from build123d import *

# Parameters (mm, degrees)
ESQUISSE1_R             = 52.5
BOSS_EXTRU_1_DEPTH      = 25
ESQUISSE2_R             = 40
ENL_V_MAT_EXTRU_1_DEPTH = 20
ESQUISSE3_R             = 22.3
BOSS_EXTRU_2_DEPTH      = 10
CHANFREIN1_SIZE         = 2
ENL_V_MAT_EXTRU_2_REACH = 77.746
ESQUISSE4_R             = 2
ESQUISSE4_R_2           = 6
ESQUISSE5_R             = 47.5
ESQUISSE5_R_2           = 42
ENL_V_MAT_EXTRU_3_DEPTH = 5
CONG_2_R                = 2.75
CHANFREIN2_SIZE         = 1
ESQUISSE6_R             = 5
ENL_V_MAT_EXTRU_4_DEPTH = 5


with BuildPart() as part:
    # Esquisse1 → Boss.-Extru.1 (new body)
    with BuildSketch(Plane(origin=(0, 0, 0), x_dir=(1, 0, 0), z_dir=(0, 1, 0))):
        with Locations(Location((0, 0, 0), (0, 0, 270))):
            Circle(ESQUISSE1_R)
    extrude(amount=BOSS_EXTRU_1_DEPTH)

    # Esquisse2 → Enlèv. mat.-Extru.1 (cut)
    with BuildSketch(Plane(origin=(0, 25, 0), x_dir=(1, 0, 0), z_dir=(0, 1, 0))):
        with Locations(Location((0, 0, 0), (0, 0, 270))):
            Circle(ESQUISSE2_R)
    extrude(amount=-ENL_V_MAT_EXTRU_1_DEPTH, mode=Mode.SUBTRACT)

    # Esquisse3 → Boss.-Extru.2 (add)
    with BuildSketch(Plane(origin=(0, 5, 0), x_dir=(1, 0, 0), z_dir=(0, 1, 0))):
        with Locations(Location((0, 0, 0), (0, 0, 270))):
            Circle(ESQUISSE3_R)
    extrude(amount=BOSS_EXTRU_2_DEPTH)

    # Chanfrein1
    chanfrein1_edges = [part.edges().sort_by_distance(p)[0] for p in [
        (0, 15, -22.3),
    ]]
    chamfer(chanfrein1_edges, length=CHANFREIN1_SIZE)

    # Esquisse4 → Enlèv. mat.-Extru.2 (cut, up to next)
    with BuildSketch(Plane(origin=(0, 15, 0), x_dir=(1, 0, 0), z_dir=(0, 1, 0)), mode=Mode.PRIVATE) as enl_v_mat_extru_2_sk1:
        with Locations(Location((0, 16, 0), (0, 0, 270))):
            Circle(ESQUISSE4_R)
    enl_v_mat_extru_2_tool1 = extrude(enl_v_mat_extru_2_sk1.sketch, amount=-ENL_V_MAT_EXTRU_2_REACH, mode=Mode.PRIVATE) & part.part
    # Esquisse4 → Enlèv. mat.-Extru.2 (cut, up to next)
    with BuildSketch(Plane(origin=(0, 15, 0), x_dir=(1, 0, 0), z_dir=(0, 1, 0)), mode=Mode.PRIVATE) as enl_v_mat_extru_2_sk2:
        with Locations(Location((13.856406461, 8, 0), (0, 0, 270))):
            Circle(ESQUISSE4_R)
    enl_v_mat_extru_2_tool2 = extrude(enl_v_mat_extru_2_sk2.sketch, amount=-ENL_V_MAT_EXTRU_2_REACH, mode=Mode.PRIVATE) & part.part
    # Esquisse4 → Enlèv. mat.-Extru.2 (cut, up to next)
    with BuildSketch(Plane(origin=(0, 15, 0), x_dir=(1, 0, 0), z_dir=(0, 1, 0)), mode=Mode.PRIVATE) as enl_v_mat_extru_2_sk3:
        with Locations(Location((13.856406461, -8, 0), (0, 0, 270))):
            Circle(ESQUISSE4_R)
    enl_v_mat_extru_2_tool3 = extrude(enl_v_mat_extru_2_sk3.sketch, amount=-ENL_V_MAT_EXTRU_2_REACH, mode=Mode.PRIVATE) & part.part
    # Esquisse4 → Enlèv. mat.-Extru.2 (cut, up to next)
    with BuildSketch(Plane(origin=(0, 15, 0), x_dir=(1, 0, 0), z_dir=(0, 1, 0)), mode=Mode.PRIVATE) as enl_v_mat_extru_2_sk4:
        with Locations(Location((0, -16, 0), (0, 0, 270))):
            Circle(ESQUISSE4_R)
    enl_v_mat_extru_2_tool4 = extrude(enl_v_mat_extru_2_sk4.sketch, amount=-ENL_V_MAT_EXTRU_2_REACH, mode=Mode.PRIVATE) & part.part
    # Esquisse4 → Enlèv. mat.-Extru.2 (cut, up to next)
    with BuildSketch(Plane(origin=(0, 15, 0), x_dir=(1, 0, 0), z_dir=(0, 1, 0)), mode=Mode.PRIVATE) as enl_v_mat_extru_2_sk5:
        with Locations(Location((-13.856406461, -8, 0), (0, 0, 270))):
            Circle(ESQUISSE4_R)
    enl_v_mat_extru_2_tool5 = extrude(enl_v_mat_extru_2_sk5.sketch, amount=-ENL_V_MAT_EXTRU_2_REACH, mode=Mode.PRIVATE) & part.part
    # Esquisse4 → Enlèv. mat.-Extru.2 (cut, up to next)
    with BuildSketch(Plane(origin=(0, 15, 0), x_dir=(1, 0, 0), z_dir=(0, 1, 0)), mode=Mode.PRIVATE) as enl_v_mat_extru_2_sk6:
        with Locations(Location((-13.856406461, 8, 0), (0, 0, 270))):
            Circle(ESQUISSE4_R)
    enl_v_mat_extru_2_tool6 = extrude(enl_v_mat_extru_2_sk6.sketch, amount=-ENL_V_MAT_EXTRU_2_REACH, mode=Mode.PRIVATE) & part.part
    # Esquisse4 → Enlèv. mat.-Extru.2 (cut, up to next)
    with BuildSketch(Plane(origin=(0, 15, 0), x_dir=(1, 0, 0), z_dir=(0, 1, 0)), mode=Mode.PRIVATE) as enl_v_mat_extru_2_sk7:
        with Locations(Location((0, 0, 0), (0, 0, 270))):
            Circle(ESQUISSE4_R_2)
    enl_v_mat_extru_2_tool7 = extrude(enl_v_mat_extru_2_sk7.sketch, amount=-ENL_V_MAT_EXTRU_2_REACH, mode=Mode.PRIVATE) & part.part
    add(enl_v_mat_extru_2_tool1.solids().sort_by_distance((0, 15, -16))[0], mode=Mode.SUBTRACT)
    add(enl_v_mat_extru_2_tool2.solids().sort_by_distance((13.856406, 15, -8))[0], mode=Mode.SUBTRACT)
    add(enl_v_mat_extru_2_tool3.solids().sort_by_distance((13.856406, 15, 8))[0], mode=Mode.SUBTRACT)
    add(enl_v_mat_extru_2_tool4.solids().sort_by_distance((0, 15, 16))[0], mode=Mode.SUBTRACT)
    add(enl_v_mat_extru_2_tool5.solids().sort_by_distance((-13.856406, 15, 8))[0], mode=Mode.SUBTRACT)
    add(enl_v_mat_extru_2_tool6.solids().sort_by_distance((-13.856406, 15, -8))[0], mode=Mode.SUBTRACT)
    add(enl_v_mat_extru_2_tool7.solids().sort_by_distance((0, 15, 0))[0], mode=Mode.SUBTRACT)

    # Esquisse5 → Enlèv. mat.-Extru.3 (cut)
    with BuildSketch(Plane(origin=(0, 25, 0), x_dir=(1, 0, 0), z_dir=(0, 1, 0))):
        with Locations(Location((0, 0, 0), (0, 0, 270))):
            Circle(ESQUISSE5_R)
        with Locations(Location((0, 0, 0), (0, 0, 270))):
            Circle(ESQUISSE5_R_2, mode=Mode.SUBTRACT)
    extrude(amount=-ENL_V_MAT_EXTRU_3_DEPTH, mode=Mode.SUBTRACT)

    # Congé2
    cong_2_edges = [part.edges().sort_by_distance(p)[0] for p in [
        (0, 20, -47.5),
        (0, 20, -42),
    ]]
    fillet(cong_2_edges, radius=CONG_2_R - 0.0001)  # a hair under: the kernel refuses the full size

    # Chanfrein2
    chanfrein2_edges = [part.edges().sort_by_distance(p)[0] for p in [
        (0, 25, -42),
    ]]
    chamfer(chanfrein2_edges, length=CHANFREIN2_SIZE)

    # Esquisse6 → Enlèv. mat.-Extru.4 (cut)
    with BuildSketch(Plane.XZ):
        with Locations(Location((0, 16, 0), (0, 0, 270))):
            Circle(ESQUISSE6_R)
        with Locations(Location((13.856406461, 8, 0), (0, 0, 270))):
            Circle(ESQUISSE6_R)
        with Locations(Location((13.856406461, -8, 0), (0, 0, 270))):
            Circle(ESQUISSE6_R)
        with Locations(Location((0, -16, 0), (0, 0, 270))):
            Circle(ESQUISSE6_R)
        with Locations(Location((-13.856406461, -8, 0), (0, 0, 270))):
            Circle(ESQUISSE6_R)
        with Locations(Location((-13.856406461, 8, 0), (0, 0, 270))):
            Circle(ESQUISSE6_R)
    extrude(amount=-ENL_V_MAT_EXTRU_4_DEPTH, mode=Mode.SUBTRACT)


solid = part.part
Here's how the part is built. I have some questions about the finished solid (model axes, mm). A direction names the side the tool comes from. Give positions to 0.01 mm unless a question says otherwise; leave off trailing zeros. Order: outer loops, then holes, each group sorted by start corner. A loop starts at its lowest first (then second) coordinate and runs counter-clockwise, first axis right, second up. Notation, with made-up numbers: (23.25, 13) -> (43.25, 13) arc R25 cw to (43.25, 26) -> close; hole circle Ø6 at (57.5, 82). An arc over 180 degrees is marked (long way). Use a Markdown table: item, result. Add a question column.
Item 1: Imagine slicing it at C-C on y = 18.5. Please give me the cut outline in (x, z).
Item 2: For faces 3 (the face through (-11, 0, -1)), 4 (the face through (-4, 15, -5)), 5 (the face through (-2.2, 5, 16.1)), which set-ups out of +Z, -Z, +X, -X, +Y, -Y let a thin tool reach every point of the face, with its end or its side?
Item 3: Will these pins go through, and if not, where does the flat tip stop? pin 1 (3.5 mm diameter, centred on x = 0, z = 16, fed in from +Y) (1 decimal); pin 2 (2 mm diameter, centred on y = 9, z = 6, fed in from -X); pin 3 (1.5 mm diameter, centred on x = -9.5, y = 15.5, fed in from +Z); pin 4 (6 mm diameter, centred on y = 21.5, z = 39.5, fed in from +X).
Item 4: I need wall thicknesses on line 1 (X direction, y = 23.3, z = 0); line 2 (X direction, y = 2.75, z = 8); line 3 (X direction, y = 13, z = 5). Which ranges of each line are inside material? Lowest first, please.
Item 5: Imagine slicing it at B-B on y = 11.75. Give the number of separate pieces and of enclosed holes in the cut face, plus the area to 3 significant figures.
Item 6: If we mould it in two halves opening along X, with no side actions, what happens to faces 1 (the face through (-46.4, 25, -11.9)), 2 (the face through (13.9, 5, 5.8))? For each: pulls with the +X half, pulls with the -X half, needs draft (parallel to the pull), parting line crosses it, or undercut.
Data:
| question | item | result |
|---|---|---|
| 1 | outline | circle Ø105 at (0, 0); hole circle Ø80 at (0, 0) |
| 2 | face 3 | +Z, -Z, +X, -X, -Y |
| 2 | face 4 | +Y |
| 2 | face 5 | -Y |
| 3 | pin 1 | passes through |
| 3 | pin 2 | stops at x = -52.26 |
| 3 | pin 3 | stops at z = 51.77 |
| 3 | pin 4 | stops at x = 37.74 |
| 4 | line 1 | x = -52.5 to -47.5, -42 to -40, 40 to 42, 47.5 to 52.5 |
| 4 | line 2 | x = -51.89 to -18.86, -8.86 to 8.86, 18.86 to 51.89 |
| 4 | line 3 | x = -52.26 to -39.69, -21.73 to -3.32, 3.32 to 21.73, 39.69 to 52.26 |
| 5 | separate pieces | 2 |
| 5 | enclosed holes | 8 |
| 5 | area | 5,010 mm² |
| 6 | face 1 | needs draft |
| 6 | face 2 | undercut |
